```python
from build123d import *

# Parameters (mm, degrees)
ESTRUSIONE_ESTRUSIONE1_DEPTH = 26
ESTRUSIONE_ESTRUSIONE2_DEPTH = 25
TAGLIO_ESTRUSIONE1_DEPTH     = 5
TAGLIO_ESTRUSIONE2_DEPTH     = 5
SCHIZZO5_R                   = 1.5
TAGLIO_ESTRUSIONE3_DEPTH     = 6.8
SCHIZZO6_R                   = 1.5
TAGLIO_ESTRUSIONE4_DEPTH     = 6.8


with BuildPart() as part:
    # Schizzo1 → Estrusione-Estrusione1 (new body)
    with BuildSketch(Plane.XY):
        Polygon((3, 0), (-3, 0), (-6, 3), (-6, 4), (-3, 4), (-3, 5.8), (3, 5.8), (3, 4), (6, 4), (6, 3), align=None)
    extrude(amount=ESTRUSIONE_ESTRUSIONE1_DEPTH)

    # Schizzo2 → Estrusione-Estrusione2 (add)
    with BuildSketch(Plane(origin=(0, 0, 0), x_dir=(1, 0, 0), z_dir=(0, 1, 0))):
        Polygon((3, 0), (6, -3), (6, -4), (3, -4), (3, -5.8), (-3, -5.8), (-3, -4), (-6, -4), (-6, -3), (-3, 0), align=None)
    extrude(amount=ESTRUSIONE_ESTRUSIONE2_DEPTH)

    # Schizzo3 → Taglio-Estrusione1 (cut)
    with BuildSketch(Plane(origin=(0, 0, 0), x_dir=(1, 0, 0), z_dir=(0, 1, 0))):
        Polygon((-3, 0), (-6, -3), (-6, 0), align=None)
        Polygon((6, -3), (6, 0), (3, 0), align=None)
    extrude(amount=TAGLIO_ESTRUSIONE1_DEPTH, mode=Mode.SUBTRACT)

    # Schizzo4 → Taglio-Estrusione2 (cut)
    with BuildSketch(Plane.XY.offset(4)):
        Polygon((-6, 3), (-3, 0), (-6, 0), align=None)
        Polygon((3, 0), (6, 0), (6, 3), align=None)
    extrude(amount=-TAGLIO_ESTRUSIONE2_DEPTH, mode=Mode.SUBTRACT)

    # Schizzo5 → Taglio-Estrusione3 (cut, through all)
    with BuildSketch(Plane.XY.offset(5.8)):
        with Locations((0, 15.4)):
            Circle(SCHIZZO5_R)
    extrude(amount=-TAGLIO_ESTRUSIONE3_DEPTH, mode=Mode.SUBTRACT)

    # Schizzo6 → Taglio-Estrusione4 (cut, through all)
    with BuildSketch(Plane(origin=(0, 5.8, 0), x_dir=(1, 0, 0), z_dir=(0, 1, 0))):
        with Locations((0, -18.3)):
            Circle(SCHIZZO6_R)
    extrude(amount=-TAGLIO_ESTRUSIONE4_DEPTH, mode=Mode.SUBTRACT)


solid = part.part
```
Design review of the part built by this model. Coordinates are the model's own, in mm. A direction names the side the tool comes from. Give positions to 0.01 mm unless a question says otherwise; leave off trailing zeros. Loops run counter-clockwise (first coordinate to the right, second up) from the corner with the lowest first, then second, coordinate; pieces in that order, holes last. Notation, with made-up numbers: M 40.25,-1 L 81.25,-1 A36 ccw 81.25,36 Z; hole C -0.5,0 d4. An arc over 180 degrees is marked long. Return JSON: item names as keys, results as strings. Group by question number.
Item 1: We need section D-D (y = 2.25). Give the boundary of the cut face in (x, z).
Item 2: We need section A-A (z = 18.3). Give the boundary of the cut face in (x, y).
Item 3: Insertion check: pin 1 Ø2.5 at (x, y) = (-5, 12) entering from +Z; pin 2 Ø1.5 at (x, z) = (3, 11) entering from +Y; pin 3 Ø1.8 at (x, y) = (0.5, 12) entering from +Z; pin 4 Ø3.5 at (x, z) = (0, 18.3) entering from -Y. Each pin has a flat end and moves straight along its axis. Give the tip position at first contact, or say it passes through.
Item 4: We need section C-C (x = 0). Give the boundary of the cut face in (y, z), and give its area (3 significant figures).
Item 5: Tool access review of faces 1 (the flat face through (-5, 2, 13)), 2 (the flat face through (4, 12, 1)), 3 (the flat face through (5, 14, 4)), 4 (the flat face through (0, 5.8, 16)), 5 (the flat face through (-5, 4, 15)): name each direction out of +Z, -Z, +X, -X, +Y, -Y from which nothing blocks a thin tool from reaching the whole face with its end or side.
Item 6: For probe 1 along Y at (x, z) = (0, 1.4); probe 2 along X at (y, z) = (3.75, 18.3); probe 3 along Y at (x, z) = (-4.5, 13), list the stretches that pass through material, from the lowest coordinate up.
Item 7: Mouldability with a two-part tool opening along X and no side actions: class faces 6 (the flat face through (3, 5, 10)), 7 (the flat face through (-3, 5, 10)), 8 (the cylindrical face through (-0.195, 16.887, 2.941)) as released by +X, released by -X, zero draft, split by the parting line, or undercut.
Output:
{
 "1": {"outline": "M -5.25,2.25 L -3,0 L 3,0 L 5.25,2.25 L 5.25,26 L -5.25,26 Z; hole C 0,18.3 d3"},
 "2": {"outline": "M -6,3 L -3,0 L -1.5,0 L -1.5,5.8 L -3,5.8 L -3,4 L -6,4 Z; M 1.5,0 L 3,0 L 6,3 L 6,4 L 3,4 L 3,5.8 L 1.5,5.8 Z"},
 "3": {"pin 1": "stops at z = 4", "pin 2": "stops at y = 5.8", "pin 3": "stops at z = 5.8", "pin 4": "stops at y = 0"},
 "4": {"outline": "M 0,0 L 13.9,0 L 13.9,5.8 L 5.8,5.8 L 5.8,16.8 L 0,16.8 Z; M 0,19.8 L 5.8,19.8 L 5.8,26 L 0,26 Z; M 16.9,0 L 25,0 L 25,5.8 L 16.9,5.8 Z", "area": "227 mm^2"},
 "5": {"face 1": "+Z, -Z, -X, -Y", "face 2": "-Z, +X, +Y, -Y", "face 3": "+Z, +X, +Y", "face 4": "+Z, +X, -X, +Y", "face 5": "+Z, -X, +Y"},
 "6": {"probe 1": "y = 0 to 13.9, 16.9 to 25", "probe 2": "x = -6 to -1.5, 1.5 to 6", "probe 3": "y = 1.5 to 4"},
 "7": {"face 6": "released by +X", "face 7": "released by -X", "face 8": "undercut"}
}
